```python
from build123d import *

# Parameters (mm, degrees)
SKETCH1_R           = 2.65
BOSS_EXTRUDE1_DEPTH = 5
CUT_EXTRUDE2_REACH  = 7
SKETCH3_R           = 2.25
FILLET1_R           = 10
SKETCH4_R           = 3.75
CUT_EXTRUDE3_DEPTH  = 1
CHAMFER1_SIZE       = 3


with BuildPart() as part:
    # Sketch1 → Boss-Extrude1 (new body)
    with BuildSketch(Plane(origin=(0, 0, 0), x_dir=(1, 0, 0), z_dir=(0, 1, 0))):
        with BuildLine():
            Line((0, 10), (40, 10))
            Line((40, 10), (40, -10))
            Line((40, -10), (0, -10))
            Line((0, -10), (-17.016791442, -5.164570129))
            Line((-17.016791442, -5.164570129), (-22.567561857, 18))
            ThreePointArc((-22.567561857, 18), (-19.742561857, 22.893043531), (-14.092561857, 22.893043531))
            Line((-14.092561857, 22.893043531), (0, 10))
        make_face()
        with Locations((-16.917561857, 18)):
            Circle(SKETCH1_R, mode=Mode.SUBTRACT)
        with Locations((-12, -0.352590699)):
            Circle(SKETCH1_R, mode=Mode.SUBTRACT)
    extrude(amount=BOSS_EXTRUDE1_DEPTH)

    # Sketch3 → Cut-Extrude2 (cut, up to next)
    with BuildSketch(Plane(origin=(0, 5, 0), x_dir=(1, 0, 0), z_dir=(0, 1, 0)), mode=Mode.PRIVATE) as cut_extrude2_sk1:
        with Locations((10, 0)):
            Circle(SKETCH3_R)
    cut_extrude2_tool1 = extrude(cut_extrude2_sk1.sketch, amount=-CUT_EXTRUDE2_REACH, mode=Mode.PRIVATE) & part.part
    add(cut_extrude2_tool1.solids().sort_by_distance((10, 5, 0))[0], mode=Mode.SUBTRACT)
    # Sketch3 → Cut-Extrude2 (cut, up to next)
    with BuildSketch(Plane(origin=(0, 5, 0), x_dir=(1, 0, 0), z_dir=(0, 1, 0)), mode=Mode.PRIVATE) as cut_extrude2_sk2:
        with Locations((30, 0)):
            Circle(SKETCH3_R)
    cut_extrude2_tool2 = extrude(cut_extrude2_sk2.sketch, amount=-CUT_EXTRUDE2_REACH, mode=Mode.PRIVATE) & part.part
    add(cut_extrude2_tool2.solids().sort_by_distance((30, 5, 0))[0], mode=Mode.SUBTRACT)

    # Fillet1
    fillet1_edges = [part.edges().sort_by_distance(p)[0] for p in [
        (-17.016791442, 2.5, 5.164570129),
    ]]
    fillet(fillet1_edges, radius=FILLET1_R)

    # Sketch4 → Cut-Extrude3 (cut)
    with BuildSketch(Plane(origin=(0, 5, 0), x_dir=(1, 0, 0), z_dir=(0, 1, 0))):
        with Locations((10, 0)):
            Circle(SKETCH4_R)
        with Locations((30, 0)):
            Circle(SKETCH4_R)
    extrude(amount=-CUT_EXTRUDE3_DEPTH, mode=Mode.SUBTRACT)

    # Chamfer1
    chamfer1_edges = [part.edges().sort_by_distance(p)[0] for p in [
        (40, 2.5, -10),
        (40, 2.5, 10),
    ]]
    chamfer(chamfer1_edges, length=CHAMFER1_SIZE)


solid = part.part
```
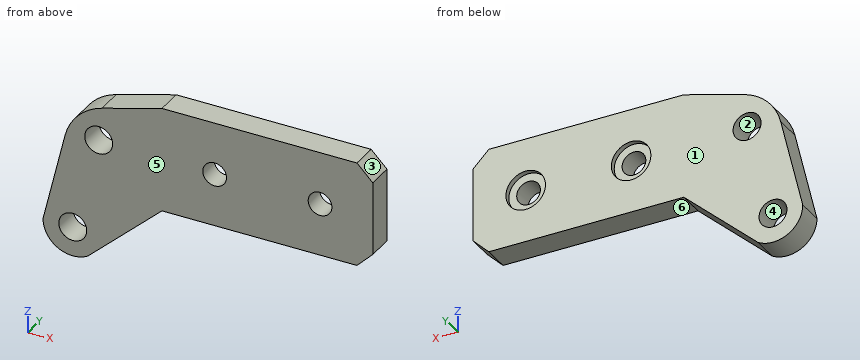
Source: CAD feature listing. Evaluate the final solid. Frame: model axes, mm. Face numbers are marked on the shaded views. A direction names the side the tool comes from. Coordinates: 2 decimals unless noted, no trailing zeros. Write each loop counter-clockwise with the first axis right and the second up, starting at its lowest first coordinate (ties: lowest second). Pieces come first, ordered by that corner, then holes. Notation, with made-up numbers: (16.25, 19.25) -> (38.25, 19.25) arc R12 ccw to (38.25, 30.25) -> close; hole circle Ø9 at (65, 81.5). An arc over 180 degrees is marked (long way). Return JSON: item names as keys, results as strings. Group by question number.
1) Mould query, pull axis X, two halves, no side actions, for the marked faces 1, 2, 3 and 4. Classes: +X half, -X half, draft (parallel to the pull), parting line (faces both ways), or undercut.
2) Section query C-C, the plane z = -19. Return loops of the section in (x, y).
3) Contact query for flat-ended pins moving along their axis: P1, Ø1, axis at y = 3.5, z = -2, coming from the -X side; P2, Ø2, axis at x = 30.5, z = -1, coming from the +Y side; P3, Ø1, axis at y = 1.5, z = -15.5, coming from the -X side. Output: stop coordinate, or through.
4) Section query D-D, the plane x = 33. Return loops of the section in (y, z), plus the area to 3 significant figures.
5) Section query B-B, the plane y = 3.05. Return loops of the section in (x, z).
6) Section query A-A, the plane x = 10. Return loops of the section in (y, z).
7) Ray query, line 1 along Z through (x, y) = (7.5, 2.75); line 2 along X through (y, z) = (3.8, -2); line 3 along Z through (x, y) = (10, 2.2). Return the intervals inside material, ascending.
8) Set-up query: the marked faces 5 and 6. Return all of +Z, -Z, +X, -X, +Y, -Y with unobstructed straight access to the full face (end or side cutting, diameter ignored); none if empty.
From the geometry:
{
 "1": {"face 1": "draft", "face 2": "undercut", "face 3": "+X half", "face 4": "undercut"},
 "2": {"outline": "(-22.48, 0) -> (-19.37, 0) -> (-19.37, 5) -> (-22.48, 5) -> close; (-14.46, 0) -> (-9.84, 0) -> (-9.84, 5) -> (-14.46, 5) -> close"},
 "3": {"P1": "x = -18.85", "P2": "through", "P3": "x = -22.09"},
 "4": {"outline": "(0, -10) -> (5, -10) -> (5, -2.25) -> (4, -2.25) -> (4, 2.25) -> (5, 2.25) -> (5, 10) -> (0, 10) -> close", "area": "95.5 mm²"},
 "5": {"outline": "(-22.57, -18) arc R5.65 ccw to (-14.09, -22.89) -> (0, -10) -> (37, -10) -> (40, -7) -> (40, 7) -> (37, 10) -> (0, 10) -> (-11.39, 6.76) arc R10 ccw to (-18.38, -0.53) -> close; hole circle Ø5.3 at (-16.92, -18); hole circle Ø5.3 at (-12, 0.35); hole circle Ø4.5 at (10, 0); hole circle Ø4.5 at (30, 0)"},
 "6": {"outline": "(0, -10) -> (5, -10) -> (5, -3.75) -> (4, -3.75) -> (4, -2.25) -> (0, -2.25) -> close; (0, 2.25) -> (4, 2.25) -> (4, 3.75) -> (5, 3.75) -> (5, 10) -> (0, 10) -> close"},
 "7": {"line 1": "-10 to 10", "line 2": "-18.73 to -13.22, -10.78 to 8.97, 11.03 to 28.97, 31.03 to 40", "line 3": "-10 to -2.25, 2.25 to 10"},
 "8": {"face 5": "+Z, -Z, +X, -X, -Y", "face 6": "-Z, +X, +Y, -Y"}
}
